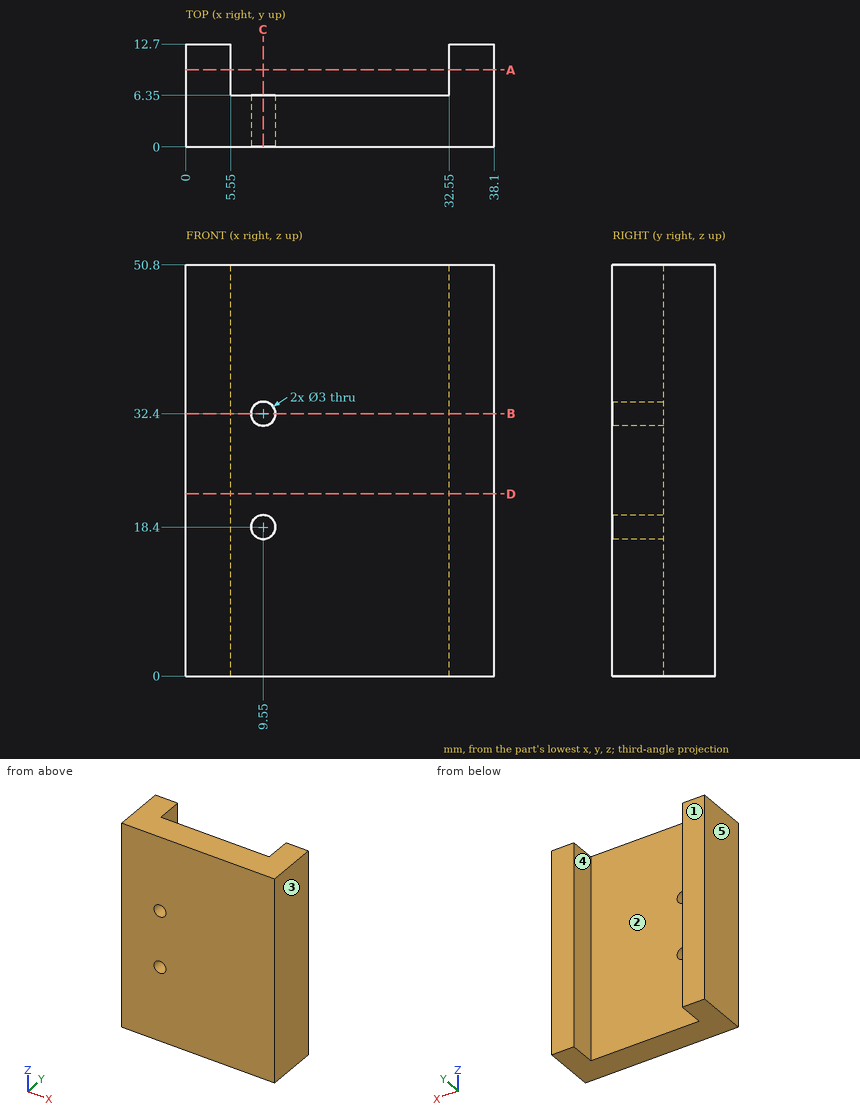
Study the drawing (mm; zero at the part's minimum x, y, z) and answer. A direction names the side the tool comes from. Round coordinates to 2 decimals unless told otherwise and drop trailing zeros. Loops run counter-clockwise (first coordinate to the right, second up) from the corner with the lowest first, then second, coordinate; pieces in that order, holes last. Notation, with made-up numbers: (63, 67.5) - (81, 67.5) arc R12 ccw to (81, 90.5) - close; hole circle Ø1 at (16.5, 64). An arc over 180 degrees is marked (long way). Use one line per item in the form item = value. Start each with the question number.
1. For a pull along X with two mould halves and no side action, classify the marked faces 1, 2 and 3 as pulls with the +X half, pulls with the -X half, needs draft (parallel to the pull), parting line crosses it, or undercut.
2. Given pin 1 Ø5 at (x, z) = (31.5, 6) entering from -Y; pin 2 Ø13.5 at (x, z) = (22, 18.5) entering from +Y; pin 3 Ø3 at (x, y) = (21, 9.5) entering from +Z, each flat-ended and moving along its own axis, determine where each tip first touches the part or whether it passes through.
3. The part is cut by section A-A on y = 9.5. Determine the outline of the cut face in (x, z), then the cut area to 3 significant figures.
4. The part is cut by section D-D on z = 22.5. Determine the outline of the cut face in (x, y), then the cut area to 3 significant figures.
5. The part is cut by section C-C on x = 9.55. Determine the outline of the cut face in (y, z), then the cut area to 3 significant figures.
6. Consider line 1 (Z direction, x = 9.55, y = 4.5); line 2 (X direction, y = 3.5, z = 32.4); line 3 (X direction, y = 10.25, z = 47). Determine where each line is inside the solid, lowest interval first. Write a range as [from, to].
7. The part is cut by section B-B on z = 32.4. Determine the outline of the cut face in (x, y).
8. A tool of negligible diameter and unlimited length cuts with its end or side. For the marked faces 4 and 5, from which of +Z, -Z, +X, -X, +Y, -Y can it reach the whole face along a straight path? Write none if from no direction.
Geometry check:
q1.face_1 = needs draft
q1.face_2 = undercut
q1.face_3 = pulls with the +X half
q2.pin_1 = 0
q2.pin_2 = 6.35
q2.pin_3 = through
q3.outline = (0, 0) - (5.55, 0) - (5.55, 50.8) - (0, 50.8) - close; (32.55, 0) - (38.1, 0) - (38.1, 50.8) - (32.55, 50.8) - close
q3.area = 564 mm^2
q4.outline = (0, 0) - (38.1, 0) - (38.1, 12.7) - (32.55, 12.7) - (32.55, 6.35) - (5.55, 6.35) - (5.55, 12.7) - (0, 12.7) - close
q4.area = 312 mm^2
q5.outline = (0, 0) - (6.35, 0) - (6.35, 16.9) - (0, 16.9) - close; (0, 19.9) - (6.35, 19.9) - (6.35, 30.9) - (0, 30.9) - close; (0, 33.9) - (6.35, 33.9) - (6.35, 50.8) - (0, 50.8) - close
q5.area = 284 mm^2
q6.line_1 = [0, 16.9], [19.9, 30.9], [33.9, 50.8]
q6.line_2 = [0, 8.05], [11.05, 38.1]
q6.line_3 = [0, 5.55], [32.55, 38.1]
q7.outline = (0, 0) - (8.05, 0) - (8.05, 6.35) - (5.55, 6.35) - (5.55, 12.7) - (0, 12.7) - close; (11.05, 0) - (38.1, 0) - (38.1, 12.7) - (32.55, 12.7) - (32.55, 6.35) - (11.05, 6.35) - close
q8.face_4 = +Z, -Z, +Y
q8.face_5 = +Z, -Z, -X, +Y, -Y
